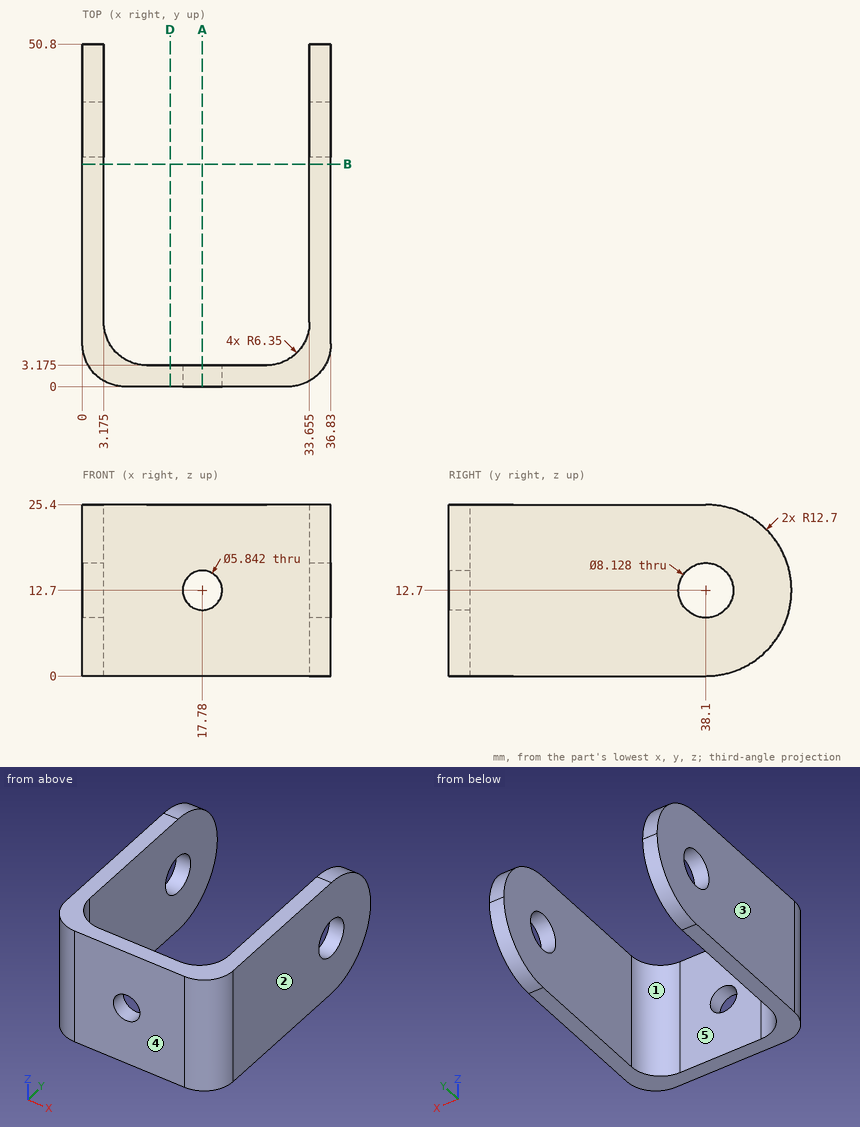
Study the drawing (mm; zero at the part's minimum x, y, z) and answer. A direction names the side the tool comes from. Round coordinates to 2 decimals unless told otherwise and drop trailing zeros. Write each loop counter-clockwise with the first axis right and the second up, starting at its lowest first coordinate (ties: lowest second). Pieces come first, ordered by that corner, then holes. Notation, with made-up numbers: (-21.75, 66.25) - (35.25, 66.25) arc R12 ccw to (35.25, 74.25) - close; hole circle Ø1 at (-10.5, 27.25). An arc over 180 degrees is marked (long way). Return JSON: item names as keys, results as strings. Group by question number.
Q1. Each of these flat-tipped pins is pushed along its axis until it touches: pin 1 Ø12 at (y, z) = (28.5, 8.5) entering from -X; pin 2 Ø4 at (x, z) = (4.5, 14.5) entering from +Y. Where does it stop, or does it pass through?
Q2. The part is cut by section A-A on x = 17.78. Write down the section's boundary in (y, z) (1 decimal).
Q3. Find the intervals of material crossed by L1, parallel to X at y = 16.5, z = 1.5 (1 decimal); L2, parallel to Z at x = 17.78, y = 2.35; L3, parallel to Y at x = 15, z = 6.75 (1 decimal), in increasing order.
Q4. The mould has two halves that part along X. Classify the marked faces 3, 4 and 5: released by +X, released by -X, zero draft, split by the parting line, or undercut.
Q5. The part is cut by section B-B on y = 33. Write down the section's boundary in (x, z) (1 decimal), then the cut area to 3 significant figures.
Q6. The part is cut by section D-D on x = 13. Write down the section's boundary in (y, z) (1 decimal).
Q7. For the marked faces 1 and 2, determine the directions among +Z, -Z, +X, -X, +Y, -Y from which every point of the face is accessible in a straight line to the end or side of a thin tool.
Solved:
{
 "1": {"pin 1": "x = 0", "pin 2": "y = 50.8"},
 "2": {"outline": "(0, 0) - (3.2, 0) - (3.2, 9.8) - (0, 9.8) - close; (0, 15.6) - (3.2, 15.6) - (3.2, 25.4) - (0, 25.4) - close"},
 "3": {"L1": "0 to 3.2, 33.7 to 36.8", "L2": "0 to 9.78, 15.62 to 25.4", "L3": "0 to 3.2"},
 "4": {"face 3": "released by -X", "face 4": "zero draft", "face 5": "undercut"},
 "5": {"outline": "(0, 0) - (3.2, 0) - (3.2, 25.4) - (0, 25.4) - close; (33.7, 0) - (36.8, 0) - (36.8, 25.4) - (33.7, 25.4) - close", "area": "161 mm²"},
 "6": {"outline": "(0, 0) - (3.2, 0) - (3.2, 25.4) - (0, 25.4) - close"},
 "7": {"face 1": "+Z, -Z, +Y", "face 2": "+Z, -Z, +X, +Y, -Y"}
}
